The drawing under review shows one solid part. Ordinate dimensions are in mm from its lowest x, y, z. A direction names the side the tool comes from. Give positions to 0.01 mm unless a question says otherwise; leave off trailing zeros. Write each loop counter-clockwise with the first axis right and the second up, starting at its lowest first coordinate (ties: lowest second). Pieces come first, ordered by that corner, then holes. Notation, with made-up numbers: (83.5, 39) -> (96.5, 39) arc R7 ccw to (96.5, 48) -> close; hole circle Ø5 at (81, 30). An arc over 180 degrees is marked (long way). Answer as a JSON object with one key per item and string values.
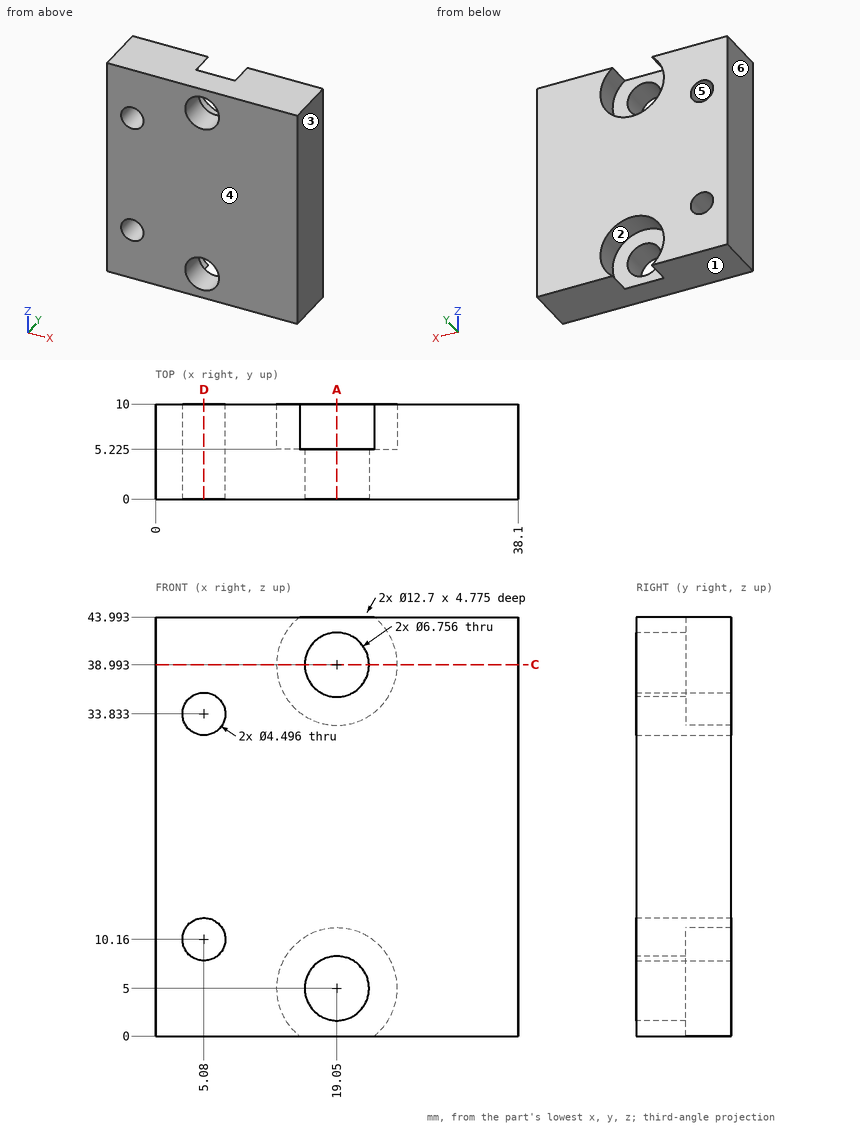
(1) We need section C-C, the plane z = 39. State the section outline as (x, y) points (1 decimal).
Here are the results:
{"outline": "(0, 0) -> (15.7, 0) -> (15.7, 5.2) -> (12.7, 5.2) -> (12.7, 10) -> (0, 10) -> close; (22.4, 0) -> (38.1, 0) -> (38.1, 10) -> (25.4, 10) -> (25.4, 5.2) -> (22.4, 5.2) -> close"}
(2) For the marked faces 1 and 2, list the 3-axis set-ups (+Z, -Z, +X, -X, +Y, -Y) from which the entire face can be reached by the end or side of a thin tool; tool diameter is ignored.
Here are the results:
{"face 1": "-Z, +X, -X, +Y, -Y", "face 2": "+Y"}
(3) The part is to be moulded in two halves that separate along X. For the marked faces 3, 4, 5 and 6, say which applies: +X half, -X half, draft (parallel to the pull), parting line (faces both ways), or undercut.
Here are the results:
{"face 3": "+X half", "face 4": "draft", "face 5": "undercut", "face 6": "-X half"}
(4) For line 1 along Z through (x, y) = (19.05, 1.8) (1 decimal); line 2 along X through (y, z) = (3.75, 10.16); line 3 along Z through (x, y) = (5.08, 3.5) (1 decimal), list the stretches that pass through material, from the lowest coordinate up.
Here are the results:
{"line 1": "z = 0 to 1.6, 8.4 to 35.6, 42.4 to 44", "line 2": "x = 0 to 2.83, 7.33 to 38.1", "line 3": "z = 0 to 7.9, 12.4 to 31.6, 36.1 to 44"}
(5) We need section A-A, the plane x = 19.05. Give the number of separate pieces and of enclosed holes in the cut face, then the cut area to 3 significant figures.
Here are the results:
{"separate pieces": "3", "enclosed holes": "0", "area": "261 mm²"}
(6) Clearance check with flat-ended pins moving along their axes: pin 1 (5.5 mm diameter, centred on x = 20, z = 6, fed in from +Y) (1 decimal); pin 2 (2 mm diameter, centred on x = 24.5, z = 23, fed in from -Y); pin 3 (4 mm diameter, centred on x = 19.05, z = 5, fed in from -Y). State where each tip first meets the part, or that it passes through.
Here are the results:
{"pin 1": "stops at y = 5.2", "pin 2": "stops at y = 0", "pin 3": "passes through"}
(7) We need section D-D, the plane x = 5.08. State the section outline as (y, z) points (1 decimal).
Here are the results:
{"outline": "(0, 0) -> (10, 0) -> (10, 7.9) -> (0, 7.9) -> close; (0, 12.4) -> (10, 12.4) -> (10, 31.6) -> (0, 31.6) -> close; (0, 36.1) -> (10, 36.1) -> (10, 44) -> (0, 44) -> close"}
